Work out the finished part from the listing and answer in its coordinate system (mm). A direction names the side the tool comes from. Round coordinates to 2 decimals unless told otherwise and drop trailing zeros. Write each loop counter-clockwise with the first axis right and the second up, starting at its lowest first coordinate (ties: lowest second). Pieces come first, ordered by that corner, then holes. Notation, with made-up numbers: M 30,85.25 L 37,85.25 A12 ccw 37,91.25 Z; hole C -35,-32.75 d11. An arc over 180 degrees is marked long. Answer in a Markdown table with one row per item.
```python
from build123d import *

# Parameters (mm, degrees)
SKETCH1_R           = 463.544695529
BOSS_EXTRUDE2_DEPTH = 76.2
EXTRUDE_THIN1_DEPTH = 76.2
SKETCH3_R           = 37.22133085
BOSS_EXTRUDE3_DEPTH = 76.2
SKETCH4_W           = 925.4067294
SKETCH4_H           = 12.7
CUT_EXTRUDE1_DEPTH  = 130.322661699
SKETCH5_R           = 50.8
CUT_EXTRUDE2_DEPTH  = 12.7
CUT_EXTRUDE3_START  = -7.62
SKETCH6_R           = 50.8
CUT_EXTRUDE3_DEPTH  = 7.62
SKETCH8_W           = 25.4
SKETCH8_H           = 21.854781484
SKETCH8_H_2         = 21.84327291
CUT_EXTRUDE4_DEPTH  = 152.4
SKETCH9_R           = 7.62
CUT_EXTRUDE5_DEPTH  = 127


# Read off the part's stored shape, not the designer's step: Extrude-Thin1
with BuildPart() as part:
    # Sketch1 → Boss-Extrude2 (new body)
    with BuildSketch(Plane(origin=(0, 0, 0), x_dir=(1, 0, 0), z_dir=(0, 1, 0))):
        with BuildLine():
            Line((533.4, -76.2), (533.4, 76.2))
            Line((533.4, 76.2), (482.762143569, 76.2))
            ThreePointArc((482.762143569, 76.2), (-488.738915233, 0), (482.762143569, -76.2))
            Line((482.762143569, -76.2), (533.4, -76.2))
        make_face()
        with Locations(Location((0, 0, 0), (0, 0, 90))):
            Circle(SKETCH1_R, mode=Mode.SUBTRACT)
    extrude(amount=BOSS_EXTRUDE2_DEPTH)

    # Extrude-Thin1 outline → Extrude-Thin1 (add)
    with BuildSketch(Plane(origin=(0, 0, 0), x_dir=(1, 0, 0), z_dir=(0, 1, 0))):
        with BuildLine():
            Line((535.94, -78.74), (535.94, 78.74))
            Line((535.94, 78.74), (484.927814167, 78.74))
            ThreePointArc((484.927814167, 78.74), (-491.278915233, 0), (484.927814167, -78.74))
            Line((484.927814167, -78.74), (535.94, -78.74))
        make_face()
        with BuildLine():
            ThreePointArc((482.762143569, -76.2), (-488.738915233, 0), (482.762143569, 76.2))
            Line((482.762143569, 76.2), (533.4, 76.2))
            Line((533.4, 76.2), (533.4, -76.2))
            Line((533.4, -76.2), (482.762143569, -76.2))
        make_face(mode=Mode.SUBTRACT)
    extrude(amount=EXTRUDE_THIN1_DEPTH)

    # Sketch3 → Boss-Extrude3 (add)
    with BuildSketch(Plane(origin=(0, 0, 0), x_dir=(1, 0, 0), z_dir=(0, 1, 0))):
        with BuildLine():
            Line((50.358749063, 37.22133085), (464.47679922, 37.22133085))
            ThreePointArc((464.47679922, 37.22133085), (463.142727121, 51.21463461), (461.387175207, 65.16133085))
            Line((461.387175207, 65.16133085), (-461.387175207, 65.16133085))
            ThreePointArc((-461.387175207, 65.16133085), (-463.142727121, 51.21463461), (-464.47679922, 37.22133085))
            Line((-464.47679922, 37.22133085), (-50.358749063, 37.22133085))
            ThreePointArc((-50.358749063, 37.22133085), (-62.62133085, 0), (-50.358749063, -37.22133085))
            Line((-50.358749063, -37.22133085), (-464.47679922, -37.22133085))
            ThreePointArc((-464.47679922, -37.22133085), (-463.142727121, -51.21463461), (-461.387175207, -65.16133085))
            Line((-461.387175207, -65.16133085), (461.387175207, -65.16133085))
            ThreePointArc((461.387175207, -65.16133085), (463.142727121, -51.21463461), (464.47679922, -37.22133085))
            Line((464.47679922, -37.22133085), (50.358749063, -37.22133085))
            ThreePointArc((50.358749063, -37.22133085), (62.62133085, 0), (50.358749063, 37.22133085))
        make_face()
        with Locations(Location((0, 0, 0), (0, 0, 90))):
            Circle(SKETCH3_R, mode=Mode.SUBTRACT)
    extrude(amount=BOSS_EXTRUDE3_DEPTH)

    # Sketch4 → Cut-Extrude1 (cut)
    with BuildSketch(Plane.XY.offset(65.16133085)):
        with Locations((-3.175550533, 38.1)):
            Rectangle(SKETCH4_W, SKETCH4_H)
    extrude(amount=-CUT_EXTRUDE1_DEPTH, mode=Mode.SUBTRACT)

    # Sketch5 → Cut-Extrude2 (cut)
    with BuildSketch(Plane(origin=(0, 76.2, 0), x_dir=(1, 0, 0), z_dir=(0, 1, 0))):
        with Locations(Location((0, 0, 0), (0, 0, 270))):
            Circle(SKETCH5_R)
    extrude(amount=-CUT_EXTRUDE2_DEPTH, mode=Mode.SUBTRACT)

    # Sketch6 → Cut-Extrude3 (cut)
    with BuildSketch(Plane.XZ.offset(CUT_EXTRUDE3_START)):
        with Locations(Location((0, 0, 0), (0, 0, 90))):
            Circle(SKETCH6_R)
    extrude(amount=CUT_EXTRUDE3_DEPTH, mode=Mode.SUBTRACT)

    # Sketch8 → Cut-Extrude4 (cut)
    with BuildSketch(Plane(origin=(535.94, 0, 0), x_dir=(0, 0, -1), z_dir=(1, 0, 0))):
        with Locations((50.038, 54.731390154)):
            Rectangle(SKETCH8_W, SKETCH8_H)
        with Locations((-50.038, 56.82595057)):
            Rectangle(SKETCH8_W, SKETCH8_H_2)
    extrude(amount=-CUT_EXTRUDE4_DEPTH, mode=Mode.SUBTRACT)

    # Sketch9 → Cut-Extrude5 (cut)
    with BuildSketch(Plane(origin=(0, 0, -65.16133085), x_dir=(-1, 0, 0), z_dir=(0, 0, -1))):
        with Locations((-431.199928215, 58.518904378)):
            Circle(SKETCH9_R)
    extrude(amount=-CUT_EXTRUDE5_DEPTH, mode=Mode.SUBTRACT)


solid = part.part
```
1. A tool of negligible diameter and unlimited length cuts with its end or side. For faces 1 (the cylindrical face through (-9.28, 37.57, 463.45)), 2 (the cylindrical face through (30.911, 3.863, -40.313)), 3 (the flat face through (511, 38, -78.74)), 4 (the flat face through (383.54, 57, 50)), from which of +Z, -Z, +X, -X, +Y, -Y can it reach the whole face along a straight path? Write none if from no direction.
Calculated:
| item | result |
|---|---|
| face 1 | +Y, -Y |
| face 2 | -Y |
| face 3 | -Z, +X, +Y, -Y |
| face 4 | +X |
2. The part is cut by section B-B (z = -212). Determine the outline of the cut face in (x, y).
Calculated:
| item | result |
|---|---|
| outline | M -443.18,0 L -412.23,0 L -412.23,76.2 L -443.18,76.2 Z; M 412.23,0 L 443.18,0 L 443.18,76.2 L 412.23,76.2 Z |
3. Given pin 1 (12.5 mm diameter, centred on x = 433.5, z = 46.5, fed in from -Y); pin 2 (11 mm diameter, centred on y = 60, z = 56.5, fed in from +X); pin 3 (23 mm diameter, centred on x = 196, y = 55, fed in from +Z); pin 4 (24.5 mm diameter, centred on x = 431.2, y = 58.52, fed in from +Z) (3 decimals), each flat-ended and moving along its own axis, determine where each tip first touches the part or whether it passes through.
Calculated:
| item | result |
|---|---|
| pin 1 | stops at y = 0 |
| pin 2 | stops at x = 383.54 |
| pin 3 | stops at z = 455.32 |
| pin 4 | stops at z = 256.585 |
4. The part is cut by section A-A (x = 0). Count the separate pieces of the cut face and the enclosed holes in it, plus the area to 3 significant figures.
Calculated:
| item | result |
|---|---|
| separate pieces | 6 |
| enclosed holes | 0 |
| area | 7,220 mm² |
5. Determine the mould class of faces 5 (the flat face through (535.94, 38, 1)), 6 (the cylindrical face through (-490.85, 37.57, -20.49)), 7 (the flat face through (461, 45.904, 50)) for opening direction Z: released by +Z, released by -Z, zero draft, split by the parting line, or undercut.
Calculated:
| item | result |
|---|---|
| face 5 | zero draft |
| face 6 | split by the parting line |
| face 7 | undercut |
6. Consider line 1 along X through (y, z) = (25, 0); line 2 along X through (y, z) = (72.25, 0); line 3 along Z through (x, y) = (-269.5, 65). Determine where each line is inside the solid, lowest interval first. Write a range as from..to.
Calculated:
| item | result |
|---|---|
| line 1 | x = -491.28..-463.54, -62.62..-37.22, 37.22..62.62, 463.54..535.94 |
| line 2 | x = -491.28..-463.54, -62.62..-50.8, 50.8..62.62, 463.54..535.94 |
| line 3 | z = -410.76..-377.15, -65.16..-37.22, 37.22..65.16, 377.15..410.76 |
7. The part is cut by section D-D (z = 101). Determine the outline of the cut face in (x, y).
Calculated:
| item | result |
|---|---|
| outline | M -480.78,0 L -452.41,0 L -452.41,76.2 L -480.78,76.2 Z; M 452.41,0 L 480.78,0 L 480.78,76.2 L 452.41,76.2 Z |
